from build123d import *

# Parameters (mm, degrees)
SKETCH_W        = 104
SKETCH_H        = 104
PAD_DEPTH       = 3
SKETCH001_W     = 104
SKETCH001_H     = 104
SKETCH001_W_2   = 100
SKETCH001_H_2   = 100
PAD001_DEPTH    = 52
CHAMFER_SIZE    = 10
SKETCH003_W     = 25
SKETCH003_H     = 20
POCKET_DEPTH    = 5
CHAMFER001_SIZE = 5
SKETCH004_W     = 12.404821
SKETCH004_H     = 9.224227
PAD002_DEPTH    = 4
SKETCH005_R     = 4
SKETCH005_R_2   = 1.4
PAD003_DEPTH    = 52
SKETCH002_R     = 2.5
POCKET001_DEPTH = 5
SKETCH006_W     = 4.492853
SKETCH006_H     = 1.837998
POCKET002_DEPTH = 25


with BuildPart() as part:
    # Sketch → Pad (new body)
    with BuildSketch(Plane.XY):
        with Locations((0.627717, 3.703031)):
            Rectangle(SKETCH_W, SKETCH_H)
    extrude(amount=PAD_DEPTH)

    # Sketch001 → Pad001 (new body)
    with BuildSketch(Plane.XY.offset(3)):
        with Locations((0.627717, 3.703031)):
            Rectangle(SKETCH001_W, SKETCH001_H)
        with Locations((0.627717, 3.703031)):
            Rectangle(SKETCH001_W_2, SKETCH001_H_2, mode=Mode.SUBTRACT)
    extrude(amount=PAD001_DEPTH)

    # Chamfer
    chamfer_edges = [part.edges().sort_by_distance(p)[0] for p in [
        (-51.372283, 55.703031, 27.5),
        (52.627717, 55.703031, 27.5),
        (-51.372283, -48.296969, 27.5),
        (52.627717, -48.296969, 27.5),
        (-49.372283, 53.703031, 29),
        (50.627717, 53.703031, 29),
        (-49.372283, -46.296969, 29),
        (50.627717, -46.296969, 29),
    ]]
    chamfer(chamfer_edges, length=CHAMFER_SIZE)

    # Sketch003 → Pocket (cut)
    with BuildSketch(Plane.XZ.offset(48.296969)):
        with Locations((0.627717, 13)):
            Rectangle(SKETCH003_W, SKETCH003_H)
    extrude(amount=-POCKET_DEPTH, mode=Mode.SUBTRACT)

    # Chamfer001
    chamfer001_edges = [part.edges().sort_by_distance(p)[0] for p in [
        (-11.872283, -47.296969, 23),
        (13.127717, -47.296969, 23),
    ]]
    chamfer(chamfer001_edges, length=CHAMFER001_SIZE)

    # Sketch004 → Pad002 (new body)
    with BuildSketch(Plane.XY.offset(3)):
        with Locations((0.308178, -40.387887)):
            Rectangle(SKETCH004_W, SKETCH004_H)
    extrude(amount=PAD002_DEPTH)

    # Sketch005 → Pad003 (new body)
    with BuildSketch(Plane.XY.offset(3)):
        with Locations((-42.073699, 46.404447)):
            Circle(SKETCH005_R)
        with Locations((-42.073699, 46.404447)):
            Circle(SKETCH005_R_2, mode=Mode.SUBTRACT)
        with Locations((43.329133, 46.404447)):
            Circle(SKETCH005_R)
        with Locations((43.329133, 46.404447)):
            Circle(SKETCH005_R_2, mode=Mode.SUBTRACT)
        with Locations((-42.073699, -38.998385)):
            Circle(SKETCH005_R)
        with Locations((-42.073699, -38.998385)):
            Circle(SKETCH005_R_2, mode=Mode.SUBTRACT)
        with Locations((43.329133, -38.998385)):
            Circle(SKETCH005_R)
        with Locations((43.329133, -38.998385)):
            Circle(SKETCH005_R_2, mode=Mode.SUBTRACT)
    extrude(amount=PAD003_DEPTH)

    # Sketch002 → Pocket001 (cut)
    with BuildSketch(Plane.XY.offset(3)):
        with Locations((-42.372283, 3.703031)):
            Circle(SKETCH002_R)
        with Locations((43.627717, 3.703031)):
            Circle(SKETCH002_R)
    extrude(amount=-POCKET001_DEPTH, mode=Mode.SUBTRACT)

    # Sketch006 → Pocket002 (cut)
    with BuildSketch(Plane.YZ.offset(6.510589)):
        with Locations((-40.668302, 4.592406)):
            Rectangle(SKETCH006_W, SKETCH006_H)
    extrude(amount=-POCKET002_DEPTH, mode=Mode.SUBTRACT)


solid = part.part
Geometry check sheet. Reference: the model listing, model coordinates, mm. A direction names the side the tool comes from. Round coordinates to 2 decimals unless told otherwise and drop trailing zeros. Order: outer loops, then holes, each group sorted by start corner. A loop starts at its lowest first (then second) coordinate and runs counter-clockwise, first axis right, second up. Notation, with made-up numbers: M 8.25,-17.75 L 42.25,-17.75 A29 ccw 42.25,11.25 Z; hole C 40.25,-28.75 d5. An arc over 180 degrees is marked long. Answer in a Markdown table with one row per item.
(1) Draft check along X on faces 1 (the face through (-15, 54, 55)), 2 (the face through (-46.3, -43.37, 27.12)), 3 (the face through (42.297, 47.351, 28.636)). Enter one of: released by +X, released by -X, zero draft, split by the parting line, or undercut.
Responses:
| item | result |
|---|---|
| face 1 | zero draft |
| face 2 | released by -X |
| face 3 | undercut |
(2) Sectioned sample at B-B, the plane x = -14. Record the cut outline in (y, z).
Responses:
| item | result |
|---|---|
| outline | M -48.3,0 L 55.7,0 L 55.7,55 L 53.7,55 L 53.7,3 L -46.3,3 L -46.3,55 L -48.3,55 Z |
(3) Scan lines: probe 1 along X at (y, z) = (-2, 6); probe 2 along Y at (x, z) = (32.5, 35.5); probe 3 along X at (y, z) = (-38, 52.5). Record each from-to range of solid material in increasing order. Write a range as from..to.
Responses:
| item | result |
|---|---|
| probe 1 | x = -51.37..-49.37, 50.63..52.63 |
| probe 2 | y = -48.3..-46.3, 53.7..55.7 |
| probe 3 | x = -51.37..-47.67, -45.95..-43.06, -41.09..-38.2, 39.46..42.35, 44.31..47.2, 48.92..52.63 |
(4) Sectioned sample at C-C, the plane z = 45. Record the cut outline in (x, y), and give its area (3 significant figures).
Responses:
| item | result |
|---|---|
| outline | M -51.37,-38.3 L -41.37,-48.3 L 42.63,-48.3 L 52.63,-38.3 L 52.63,45.7 L 42.63,55.7 L -41.37,55.7 L -51.37,45.7 Z; hole M -49.37,-36.3 L -46.02,-39.65 A4 cw long -42.72,-42.95 L -39.37,-46.3 L 40.63,-46.3 L 43.98,-42.95 A4 cw long 47.28,-39.65 L 50.63,-36.3 L 50.63,43.7 L 47.28,47.05 A4 cw long 43.98,50.35 L 40.63,53.7 L -39.37,53.7 L -42.72,50.35 A4 cw long -46.02,47.05 L -49.37,43.7 Z; hole C -42.07,-39 d2.8; hole C -42.07,46.4 d2.8; hole C 43.33,-39 d2.8; hole C 43.33,46.4 d2.8 |
| area | 983 mm² |
(5) Sectioned sample at A-A, the plane y = 17.5. Record the cut outline in (x, z), and give its area (3 significant figures).
Responses:
| item | result |
|---|---|
| outline | M -51.37,0 L 52.63,0 L 52.63,55 L 50.63,55 L 50.63,3 L -49.37,3 L -49.37,55 L -51.37,55 Z |
| area | 520 mm² |
(6) Tool access check on faces 4 (the face through (0, -35.776, 5)), 5 (the face through (0, -41, 3.673)), 6 (the face through (10.663, -47.311, 20.465)). Record the directions out of +Z, -Z, +X, -X, +Y, -Y that give a thin tool (end or side, any length) a straight path to the whole face; none if there is none.
Responses:
| item | result |
|---|---|
| face 4 | +Z |
| face 5 | none |
| face 6 | -Y |
(7) Go/stop test with flat-tipped pins: P1, Ø10, axis at x = 2, y = -39.5, coming from the +Z side; P2, Ø8, axis at x = 28, y = -0.5, coming from the +Z side; P3, Ø1.5, axis at x = 0, z = 4.5, coming from the -Y side. Record where each tip stops, or that it passes through.
Responses:
| item | result |
|---|---|
| P1 | stops at z = 7 |
| P2 | stops at z = 3 |
| P3 | stops at y = -45 |
(8) Sectioned sample at D-D, the plane z = 14. State how many separate pieces and enclosed holes the cut face has, and give its area (3 significant figures).
Responses:
| item | result |
|---|---|
| separate pieces | 1 |
| enclosed holes | 4 |
| area | 933 mm² |
